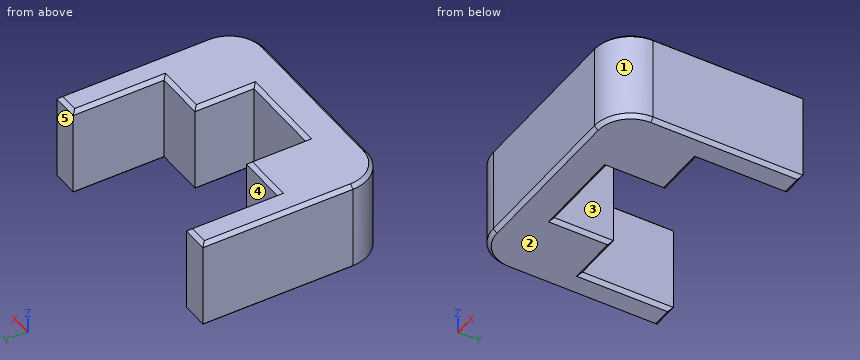
Autodesk Fusion 360 part; units mm, degrees
sketch "Sketch1" plane through (0, 0, 0) normal (0, 0, 1) x (1, 0, 0) in component "rail_installation_guide_center_x2"
  line L0 (0, -6.2924) -> (-4.6, -6.2924)
  line L1 (-4.6, -6.2924) -> (-4.6, 0.2076)
  line L2 (-4.6, 0.2076) -> (-10.1, 0.2076)
  line L3 (-10.1, 0.2076) -> (-10.1, 10.2076)
  line L4 (-10.1, 10.2076) -> (-13, 10.2076)
  line L5 (-13, 10.2076) -> (-13, -10.2924)
  line L6 (-13, -10.2924) -> (0, -10.2924)
  line L7 (0, -13) -> (0, 13) construction
  line L8 (0, -6.2924) -> (4.6, -6.2924)
  line L9 (4.6, -6.2924) -> (4.6, 0.2076)
  line L10 (4.6, 0.2076) -> (10.1, 0.2076)
  line L11 (10.1, 0.2076) -> (10.1, 10.2076)
  line L12 (10.1, 10.2076) -> (13, 10.2076)
  line L13 (13, 10.2076) -> (13, -10.2924)
  line L14 (13, -10.2924) -> (0, -10.2924)
  dimension "d9" = 4.6
  dimension "d10" = 6.5
  dimension "d11" = 10
  dimension "d13" = 2.9
  dimension "d14" = 4
  dimension "d15" = 10.1
extrude "Extrude1" add sketch "Sketch1" along normal mid plane 10 in component "rail_installation_guide_center_x2"
fillet "Fillet1" radius 4 2 edges at (-13, -10.2924, 0) (13, -10.2924, 0) in component "rail_installation_guide_center_x2"
chamfer "Chamfer1" distance 0.4 angle 45 28 edges at (-13, 1.9576, 5) (-11.8284, -9.1208, 5) (0, -10.2924, 5) (11.8284, -9.1208, 5) (13, 1.9576, 5) (-11.55, 10.2076, 5) (-10.1, 5.2076, 5) (-7.35, 0.2076, 5) (-4.6, -3.0424, 5) (0, -6.2924, 5) (4.6, -3.0424, 5) (7.35, 0.2076, 5) (10.1, 5.2076, 5) (11.55, 10.2076, 5) (11.55, 10.2076, -5) (13, 1.9576, -5) (11.8284, -9.1208, -5) (0, -10.2924, -5) (-11.8284, -9.1208, -5) (-13, 1.9576, -5) (-11.55, 10.2076, -5) (-10.1, 5.2076, -5) (-7.35, 0.2076, -5) (-4.6, -3.0424, -5) (0, -6.2924, -5) (4.6, -3.0424, -5) (7.35, 0.2076, -5) (10.1, 5.2076, -5) in component "rail_installation_guide_center_x2"
component "rail_installation_guide_center_x2" placed x (1, 0, 0) y (0, 1, 0) z (0, 0, 1) at (0, 0, 0)
equation "rail_width = 9.0 mm"
equation "tolerance = 0.2 mm"
equation "extrusion_width = 20.00 mm"
equation "arm_length = 10 mm"
equation "rail_depth = 6.5 mm"
equation "tool_thickness = 4 mm"
equation "corner_fillet = 4 mm"
equation "chamfer = 0.4 mm"
equation "d9 = ( rail_width + tolerance ) / 2"
equation "d10 = rail_depth"
equation "d11 = arm_length"
equation "arm_width = 2.9 mm"
equation "d13 = arm_width"
equation "d14 = tool_thickness"
equation "d15 = ( extrusion_width + tolerance ) / 2"
equation "d16 = tool_width / 2"
equation "tool_width = 10 mm"
equation "d20 = corner_fillet"
equation "d21 = chamfer"
Could you check a few things on this model? Use its own coordinates, in mm. Face numbers are marked on the shaded views. A direction names the side the tool comes from. Coordinates: 2 decimals unless noted, no trailing zeros. Order: outer loops, then holes, each group sorted by start corner. A loop starts at its lowest first (then second) coordinate and runs counter-clockwise, first axis right, second up. Notation, with made-up numbers: M -7,32 L 6,32 A24 ccw 6,62 Z; hole C -3,36.5 d1. An arc over 180 degrees is marked long. Use one line per item in the form item = value. Start each with the question number.
1. We'd pull the mould along X, two halves only. Please class the marked faces 1, 2 and 3: +X half, -X half, draft (parallel to the pull), parting line (faces both ways), or undercut.
2. For pin 1 (3 mm diameter, centred on x = 7, z = 0, fed in from +Y), with a flat end and sliding along its axis, tell me the tip position at first contact or that it passes through.
3. Suppose I cut it at D-D on y = -3.5. Write out the boundary of the cut face in (x, z).
4. On a 3-axis mill with a long thin cutter (end or side, diameter ignored), from which of +Z, -Z, +X, -X, +Y, -Y can I reach the whole of each face in a straight line? I mean the marked faces 4 and 5. Say none if no direction works.
5. Suppose I cut it at C-C on x = -1. Write out the boundary of the cut face in (y, z).
6. Suppose I cut it at A-A on y = 5.5. Write out the boundary of the cut face in (x, z).
7. Please list where these lines run through material, in increasing order: line 1 (X direction, y = -0.75, z = 3); line 2 (X direction, y = 6.5, z = -1.5); line 3 (Y direction, x = 9, z = 3.75).
8. Suppose I cut it at B-B on z = -4. Write out the boundary of the cut face in (x, y).
Geometry says:
q1.face_1 = +X half
q1.face_2 = draft
q1.face_3 = undercut
q2.pin_1 = 0.21
q3.outline = M -13,-4.6 L -12.6,-5 L -5,-5 L -4.6,-4.6 L -4.6,4.6 L -5,5 L -12.6,5 L -13,4.6 Z; M 4.6,-4.6 L 5,-5 L 12.6,-5 L 13,-4.6 L 13,4.6 L 12.6,5 L 5,5 L 4.6,4.6 Z
q4.face_4 = +Z, -Z, +Y
q4.face_5 = +Z, -Z, +X, -X, +Y
q5.outline = M -10.29,-4.6 L -9.89,-5 L -6.69,-5 L -6.29,-4.6 L -6.29,4.6 L -6.69,5 L -9.89,5 L -10.29,4.6 Z
q6.outline = M -13,-4.6 L -12.6,-5 L -10.5,-5 L -10.1,-4.6 L -10.1,4.6 L -10.5,5 L -12.6,5 L -13,4.6 Z; M 10.1,-4.6 L 10.5,-5 L 12.6,-5 L 13,-4.6 L 13,4.6 L 12.6,5 L 10.5,5 L 10.1,4.6 Z
q7.line_1 = -13 to -4.6, 4.6 to 13
q7.line_2 = -13 to -10.1, 10.1 to 13
q7.line_3 = -10.29 to 0.21
q8.outline = M -13,-6.29 A4 ccw -9,-10.29 L 9,-10.29 A4 ccw 13,-6.29 L 13,10.21 L 10.1,10.21 L 10.1,0.21 L 4.6,0.21 L 4.6,-6.29 L -4.6,-6.29 L -4.6,0.21 L -10.1,0.21 L -10.1,10.21 L -13,10.21 Z
